```python
from build123d import *

# Parameters (mm, degrees)
SKETCH1_W                 = 42.3
SKETCH1_H                 = 42.3
BOSS_EXTRUDE1_DEPTH       = 40.5
M3X0_5_TAPPED_HOLE2_D     = 2.5
M3X0_5_TAPPED_HOLE2_DEPTH = 6
M3X0_5_TAPPED_HOLE2_TIP   = 0.751075774
CHAMFER1_SIZE             = 5
SKETCH2_R                 = 11
BOSS_EXTRUDE2_DEPTH       = 2
SKETCH3_R                 = 2.5
BOSS_EXTRUDE3_DEPTH       = 23
CHAMFER2_SIZE             = 0.25
CUT_EXTRUDE1_DEPTH        = 71.191844256
CUT_EXTRUDE1_DEPTH_BACK   = 71.191844256
SKETCH7_W                 = 0.5
SKETCH7_H                 = 18
SKETCH4_W                 = 16
SKETCH4_H                 = 9.6
BOSS_EXTRUDE4_DEPTH       = 7


with BuildPart() as part:
    # Sketch1 → Boss-Extrude1 (new body)
    with BuildSketch(Plane(origin=(0, 0, 0), x_dir=(1, 0, 0), z_dir=(0, 1, 0))):
        Rectangle(SKETCH1_W, SKETCH1_H)
    extrude(amount=BOSS_EXTRUDE1_DEPTH)

    # M3x0.5 Tapped Hole2
    with Locations(Plane(origin=(0, 40.5, 0), x_dir=(1, 0, 0), z_dir=(0, 1, 0))):
        with Locations((0, 0), (15.5, 15.5), (-15.5, -15.5), (-15.5, 15.5), (15.5, -15.5)):
            Hole(M3X0_5_TAPPED_HOLE2_D / 2, depth=M3X0_5_TAPPED_HOLE2_DEPTH)
            with Locations((0, 0, -(M3X0_5_TAPPED_HOLE2_DEPTH + M3X0_5_TAPPED_HOLE2_TIP / 2))):  # 118° drill point
                Cone(0, M3X0_5_TAPPED_HOLE2_D / 2, M3X0_5_TAPPED_HOLE2_TIP, mode=Mode.SUBTRACT)

    # Chamfer1
    chamfer1_edges = [part.edges().sort_by_distance(p)[0] for p in [
        (21.15, 20.25, 21.15),
        (-21.15, 20.25, 21.15),
        (-21.15, 20.25, -21.15),
        (21.15, 20.25, -21.15),
    ]]
    chamfer(chamfer1_edges, length=CHAMFER1_SIZE)

    # Sketch2 → Boss-Extrude2 (add)
    with BuildSketch(Plane(origin=(0, 40.5, 0), x_dir=(1, 0, 0), z_dir=(0, 1, 0))):
        with Locations(Location((0, 0, 0), (0, 0, 270))):
            Circle(SKETCH2_R)
    extrude(amount=BOSS_EXTRUDE2_DEPTH)

    # Sketch3 → Boss-Extrude3 (add)
    with BuildSketch(Plane(origin=(0, 40.5, 0), x_dir=(1, 0, 0), z_dir=(0, 1, 0))):
        with Locations(Location((0, 0, 0), (0, 0, 270))):
            Circle(SKETCH3_R)
    extrude(amount=BOSS_EXTRUDE3_DEPTH)

    # Chamfer2
    chamfer2_edges = [part.edges().sort_by_distance(p)[0] for p in [
        (0, 63.5, -2.5),
    ]]
    chamfer(chamfer2_edges, length=CHAMFER2_SIZE)

    # Sketch7 → Cut-Extrude1 (cut, two sides: drawn at the far end of the back side and taken through both)
    with BuildSketch(Plane.XY.offset(-CUT_EXTRUDE1_DEPTH_BACK)):
        with Locations((-2.25, 54.5)):
            Rectangle(SKETCH7_W, SKETCH7_H)
    extrude(amount=CUT_EXTRUDE1_DEPTH + CUT_EXTRUDE1_DEPTH_BACK, mode=Mode.SUBTRACT)

    # Sketch4 → Boss-Extrude4 (add)
    with BuildSketch(Plane(origin=(21.15, 0, 0), x_dir=(0, 0, -1), z_dir=(1, 0, 0))):
        with Locations((0, 4.8)):
            Rectangle(SKETCH4_W, SKETCH4_H)
    extrude(amount=BOSS_EXTRUDE4_DEPTH)


solid = part.part
```
Model file for the job. Use its own axes, mm. A direction names the side the tool comes from. Give positions to 0.01 mm unless a question says otherwise; leave off trailing zeros. Order: outer loops, then holes, each group sorted by start corner. A loop starts at its lowest first (then second) coordinate and runs counter-clockwise, first axis right, second up.
1) Pin check, flat tips, straight feed: pin 1 (3 mm diameter, centred on x = 15.5, z = 15.5, fed in from +Y); pin 2 (3.5 mm diameter, centred on y = 54.5, z = 0, fed in from -X); pin 3 (2 mm diameter, centred on x = -15.5, z = -15.5, fed in from +Y). Stop position of each tip, or through.
2) Mould opens along X. For faces 1 (the flat face through (-21.15, 20, 0)), 2 (the cylindrical face through (-14.579, 37.458, -16.345)), 3 (the flat face through (18.7, 20, 18.6)), 4 (the flat face through (25, 5, -8)) say: +X half, -X half, draft (parallel to the pull), parting line (faces both ways), or undercut.
3) Saw through at B-B, the plane z = 17.5. Write the cut outline in (x, y), then the cut area to 3 significant figures.
4) 3-axis set-ups, long thin cutter, end or side, ignore diameter. For faces 5 (the flat face through (28.15, 5, 0)), 6 (the flat face through (-2, 54, 0)), 7 (the cylindrical face through (0.27, 37.46, 1.22)), 8 (the cylindrical face through (-15.34, 37.46, 14.26)): which of +Z, -Z, +X, -X, +Y, -Y reach the whole face in a straight line?
5) Saw through at A-A, the plane y = 26.5. Write the cut outline in (x, z).
6) Wall check: probe 1 along X at (y, z) = (38.05, 15.5); probe 2 along Z at (x, y) = (0, 38). Give the ranges that are in metal, low to high.
Computed:
1. pin 1: stops at y = 40.5
1. pin 2: stops at x = -2
1. pin 3: stops at y = 34.35
2. face 1: -X half
2. face 2: undercut
2. face 3: +X half
2. face 4: draft
3. outline: (-19.8, 0) - (19.8, 0) - (19.8, 40.5) - (-19.8, 40.5) - close
3. area: 1,600 mm2
4. face 5: +Z, -Z, +X, +Y, -Y
4. face 6: +Z, -Z, -X, +Y
4. face 7: none
4. face 8: +Y
5. outline: (-21.15, -16.15) - (-16.15, -21.15) - (16.15, -21.15) - (21.15, -16.15) - (21.15, 16.15) - (16.15, 21.15) - (-16.15, 21.15) - (-21.15, 16.15) - close
6. probe 1: x = -21.15 to -16.75, -14.25 to 14.25, 16.75 to 21.15
6. probe 2: z = -21.15 to -1.25, 1.25 to 21.15
